Work out the finished part from the listing and answer in its coordinate system (mm). Face numbers are marked on the shaded views. Round coordinates to 2 decimals unless told otherwise and drop trailing zeros. Order: outer loops, then holes, each group sorted by start corner. A loop starts at its lowest first (then second) coordinate and runs counter-clockwise, first axis right, second up. Notation, with made-up numbers: (35, 23) - (65, 23) arc R15 cw to (65, 51) - close; hole circle Ø4 at (51, 87). An arc over 180 degrees is marked (long way). Answer in a Markdown table with one row per item.
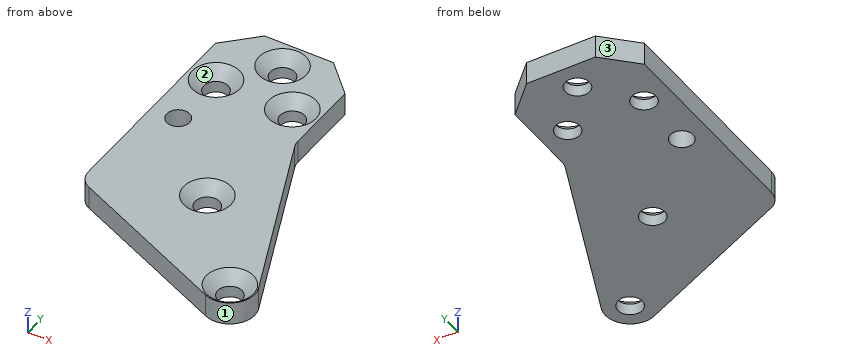
from build123d import *

# Parameters (mm, degrees)
SKETCH_1_R      = 1.5
SKETCH_1_R_2    = 1.6
EXTRUDE_1_DEPTH = 1.5
CHAMFER_1_SIZE  = 1.5
FILLET_1_R      = 2.5
CHAMFER_2_SIZE  = 4


with BuildPart() as part:
    # 草图1 → 凸台-拉伸1 (new, symmetric)
    with BuildSketch(Plane.XY):
        with BuildLine():
            Line((-3.5, 17.5), (-3.5, -15))
            Line((-3.5, -15), (19.171710101, -25.152700357))
            ThreePointArc((19.171710101, -25.152700357), (22.768840587, -24.513519167), (23.498822385, -20.933710945))
            Line((23.498822385, -20.933710945), (13.5, 3))
            Line((13.5, 3), (13.5, 17.5))
            Line((13.5, 17.5), (-3.5, 17.5))
        make_face()
        Circle(SKETCH_1_R, mode=Mode.SUBTRACT)
        with Locations((10, -10)):
            Circle(SKETCH_1_R_2, mode=Mode.SUBTRACT)
        with Locations((20.5, -22.186533479)):
            Circle(SKETCH_1_R_2, mode=Mode.SUBTRACT)
        with Locations((0, 8)):
            Circle(SKETCH_1_R_2, mode=Mode.SUBTRACT)
        with Locations((10, 8)):
            Circle(SKETCH_1_R_2, mode=Mode.SUBTRACT)
        with Locations((5, 14)):
            Circle(SKETCH_1_R_2, mode=Mode.SUBTRACT)
    extrude(amount=EXTRUDE_1_DEPTH, both=True)

    # 倒角1
    chamfer_1_edges = [part.edges().sort_by_distance(p)[0] for p in [
        (8.4, -10, 1.5),
        (18.9, -22.186533479, 1.5),
        (-1.6, 8, 1.5),
        (8.4, 8, 1.5),
        (3.4, 14, 1.5),
    ]]
    chamfer(chamfer_1_edges, length=CHAMFER_1_SIZE)

    # 圆角1
    fillet_1_edges = [part.edges().sort_by_distance(p)[0] for p in [
        (13.5, 3, 0),
        (-3.5, -15, 0),
    ]]
    fillet(fillet_1_edges, radius=FILLET_1_R)

    # 倒角2
    chamfer_2_edges = [part.edges().sort_by_distance(p)[0] for p in [
        (13.5, 17.5, 0),
        (-3.5, 17.5, 0),
    ]]
    chamfer(chamfer_2_edges, length=CHAMFER_2_SIZE)


solid = part.part
1) Find section C-C, the plane x = 20.5. Give the vertices of the cut face in (y, z), then the cut area to 3 significant figures.
Filled in:
| item | result |
|---|---|
| outline | (-25.44, -1.5) - (-23.79, -1.5) - (-23.79, 0) - (-25.29, 1.5) - (-25.44, 1.5) - close; (-20.59, -1.5) - (-13.76, -1.5) - (-13.76, 1.5) - (-19.09, 1.5) - (-20.59, 0) - close |
| area | 23.2 mm^2 |
2) Find the intervals of material crossed by probe 1 along Y at (x, z) = (0, -1.2); probe 2 along Y at (x, z) = (-1, -0.5); probe 3 along X at (y, z) = (10.5, 1.2), in increasing order. Write a range as from..to.
Filled in:
| item | result |
|---|---|
| probe 1 | y = -16.57..-1.5, 1.5..6.4, 9.6..17 |
| probe 2 | y = -16.12..-1.12, 1.12..6.75, 9.25..16 |
| probe 3 | x = -3.5..-1.26, 1.26..8.74, 11.26..13.5 |
3) Find section A-A, the plane y = 8. Give the vertices of the cut face in (x, z), then the cut area to 3 significant figures.
Filled in:
| item | result |
|---|---|
| outline | (-3.5, -1.5) - (-1.6, -1.5) - (-1.6, 0) - (-3.1, 1.5) - (-3.5, 1.5) - close; (1.6, -1.5) - (8.4, -1.5) - (8.4, 0) - (6.9, 1.5) - (3.1, 1.5) - (1.6, 0) - close; (11.6, -1.5) - (13.5, -1.5) - (13.5, 1.5) - (13.1, 1.5) - (11.6, 0) - close |
| area | 27.3 mm^2 |
4) Each of these flat-tipped pins is pushed along its axis until it touches: pin 1 (2.5 mm diameter, centred on x = 5, y = 14, fed in from +Z); pin 2 (1 mm diameter, centred on x = 2, y = 9.5, fed in from +Z); pin 3 (4 mm diameter, centred on x = 20.5, y = -22.19, fed in from +Z); pin 4 (5 mm diameter, centred on x = 10, y = -10, fed in from +Z). Where does it stop, or does it pass through?
Filled in:
| item | result |
|---|---|
| pin 1 | passes through |
| pin 2 | stops at z = 1.4 |
| pin 3 | stops at z = 0.4 |
| pin 4 | stops at z = 0.9 |
5) Find section D-D, the plane x = 10. Give the vertices of the cut face in (y, z), then the cut area to 3 significant figures.
Filled in:
| item | result |
|---|---|
| outline | (-21.05, -1.5) - (-11.6, -1.5) - (-11.6, 0) - (-13.1, 1.5) - (-21.05, 1.5) - close; (-8.4, -1.5) - (6.4, -1.5) - (6.4, 0) - (4.9, 1.5) - (-6.9, 1.5) - (-8.4, 0) - close; (9.6, -1.5) - (17, -1.5) - (17, 1.5) - (11.1, 1.5) - (9.6, 0) - close |
| area | 90.4 mm^2 |
6) The mould has two halves that part along Y. Classify the marked faces 1, 2 and 3: released by +Y, released by -Y, zero draft, split by the parting line, or undercut.
Filled in:
| item | result |
|---|---|
| face 1 | split by the parting line |
| face 2 | undercut |
| face 3 | released by +Y |
7) Find section B-B, the plane y = 14. Give the vertices of the cut face in (x, z).
Filled in:
| item | result |
|---|---|
| outline | (-3, -1.5) - (3.4, -1.5) - (3.4, 0) - (1.9, 1.5) - (-3, 1.5) - close; (6.6, -1.5) - (13, -1.5) - (13, 1.5) - (8.1, 1.5) - (6.6, 0) - close |
